```python
from build123d import *

# Parameters (mm, degrees)
SKETCH2_W           = 30
SKETCH2_H           = 90
SKETCH2_R           = 3
BOSS_EXTRUDE1_DEPTH = 3
SKETCH3_R           = 76.2
BOSS_EXTRUDE2_DEPTH = 3
SKETCH4_W           = 40
SKETCH4_H           = 10
BOSS_EXTRUDE3_DEPTH = 3
SKETCH5_W           = 40
SKETCH5_H           = 10
BOSS_EXTRUDE4_DEPTH = 3


with BuildPart() as part:
    # Sketch2 → Boss-Extrude1 (new body)
    with BuildSketch(Plane.XY):
        Rectangle(SKETCH2_W, SKETCH2_H)
        with Locations((-8.25, 20)):
            Circle(SKETCH2_R, mode=Mode.SUBTRACT)
        with Locations((8.25, 20)):
            Circle(SKETCH2_R, mode=Mode.SUBTRACT)
        with Locations((-8.25, -35)):
            Circle(SKETCH2_R, mode=Mode.SUBTRACT)
        with Locations((8.25, -35)):
            Circle(SKETCH2_R, mode=Mode.SUBTRACT)
    extrude(amount=BOSS_EXTRUDE1_DEPTH)

    # Sketch3 → Boss-Extrude2 (add)
    with BuildSketch(Plane(origin=(0, 45, 0), x_dir=(1, 0, 0), z_dir=(0, 1, 0))):
        with Locations(Location((0, -1.855318654, 0), (0, 0, 270))):
            Circle(SKETCH3_R)
    extrude(amount=BOSS_EXTRUDE2_DEPTH)

    # Sketch4 → Boss-Extrude3 (add)
    with BuildSketch(Plane(origin=(15, 0, 0), x_dir=(0, 0, -1), z_dir=(1, 0, 0))):
        with Locations((-1.5, 40)):
            Rectangle(SKETCH4_W, SKETCH4_H)
    extrude(amount=-BOSS_EXTRUDE3_DEPTH)

    # Sketch5 → Boss-Extrude4 (add)
    with BuildSketch(Plane.ZY.offset(15)):
        with Locations((1.5, 40)):
            Rectangle(SKETCH5_W, SKETCH5_H)
    extrude(amount=-BOSS_EXTRUDE4_DEPTH)


solid = part.part
```
For this review, take the finished solid that the model builds, in its own axes (mm). A direction names the side the tool comes from. Round coordinates to 2 decimals unless told otherwise and drop trailing zeros. Write each loop counter-clockwise with the first axis right and the second up, starting at its lowest first coordinate (ties: lowest second). Pieces come first, ordered by that corner, then holes. Notation, with made-up numbers: (11.25, 36.5) -> (26.25, 36.5) arc R21 ccw to (26.25, 44.5) -> close; hole circle Ø10 at (-1.5, 24). An arc over 180 degrees is marked (long way). One line per question, with ' | ' between items. Start each with the question number.
(1) Mouldability with a two-part tool opening along Y and no side actions: class faces 5 (the face through (1, 48, 1)), 6 (the face through (9.86, -32.47, 1.48)), 7 (the face through (0, 1, 3)) as released by +Y, released by -Y, zero draft, split by the parting line, or undercut.
(2) Tool access review of faces 1 (the face through (15, 27, 2)), 2 (the face through (-15, 27, 1)), 3 (the face through (12, 40, -9)), 4 (the face through (12, 40, 12)): name each direction out of +Z, -Z, +X, -X, +Y, -Y from which nothing blocks a thin tool from reaching the whole face with its end or side.
(3) Add section A-A, the plane y = -35. Write out the cut boundary in (x, z), plus the area to 3 significant figures.
(4) For line 1 along Y through (x, z) = (-8, 1); line 2 along Z through (x, y) = (-0.5, 24); line 3 along Y through (x, z) = (62, 9), list the stretches that pass through material, from the lowest coordinate up. Write a range as from..to.
(5) Add section C-C, the plane z = 12. Write out the cut boundary in (x, y), plus the area to 3 significant figures.
(6) Add section D-D, the plane y = 14.5. Write out the cut boundary in (x, z), plus the area to 3 significant figures.
(7) Add section B-B, the plane x = -8.25. Write out the cut boundary in (y, z), plus the area to 3 significant figures.
(8) Insertion check: P1, Ø20, axis at y = 11, z = 4, coming from the -X side; P2, Ø11, axis at y = 41.5, z = 15.5, coming from the +X side; P3, Ø3.5, axis at x = 13, z = -12.5, coming from the -Y side. Each pin has a flat end and moves straight along its axis. Give the tip position at first contact, or say it passes through.
Answer list:
1) face 5: released by +Y | face 6: undercut | face 7: zero draft
2) face 1: +Z, -Z, +X, -Y | face 2: +Z, -Z, -X, -Y | face 3: -Z, -Y | face 4: +Z, -Y
3) outline: (-15, 0) -> (-11.25, 0) -> (-11.25, 3) -> (-15, 3) -> close; (-5.25, 0) -> (5.25, 0) -> (5.25, 3) -> (-5.25, 3) -> close; (11.25, 0) -> (15, 0) -> (15, 3) -> (11.25, 3) -> close | area: 54.0 mm²
4) line 1: -45..-37.99, -32.01..17.01, 22.99..48 | line 2: 0..3 | line 3: 45..48
5) outline: (-75.52, 45) -> (-15, 45) -> (-15, 35) -> (-12, 35) -> (-12, 45) -> (12, 45) -> (12, 35) -> (15, 35) -> (15, 45) -> (75.52, 45) -> (75.52, 48) -> (-75.52, 48) -> close | area: 513 mm²
6) outline: (-15, 0) -> (15, 0) -> (15, 3) -> (-15, 3) -> close | area: 90.0 mm²
7) outline: (-45, 0) -> (-38, 0) -> (-38, 3) -> (-45, 3) -> close; (-32, 0) -> (17, 0) -> (17, 3) -> (-32, 3) -> close; (23, 0) -> (45, 0) -> (45, -73.9) -> (48, -73.9) -> (48, 77.61) -> (45, 77.61) -> (45, 3) -> (23, 3) -> close | area: 689 mm²
8) P1: x = -15 | P2: x = 75.62 | P3: y = 35
